Could you check a few things on this model? Use its own coordinates, in mm. A direction names the side the tool comes from. Give positions to 0.01 mm unless a question says otherwise; leave off trailing zeros. Write each loop counter-clockwise with the first axis right and the second up, starting at its lowest first coordinate (ties: lowest second). Pieces come first, ordered by that corner, then holes. Notation, with made-up numbers: (-2.75, 38) -> (10.25, 38) arc R16 ccw to (10.25, 64) -> close; hole circle Ø5 at (-9, 2.25). An arc over 180 degrees is marked (long way). One line per question, with ' | ' between items.
from build123d import *

# Parameters (mm, degrees)
F0_W     = 5
F0_H     = 5
F1_DEPTH = 5
F0_W_2   = 45
F0_W_3   = 40
F0_H_2   = 40
F2_DEPTH = 1


# Not quite as in the source:
# - a feature of the source that left no trace in its solid (it failed there, or was rolled back) is left out


with BuildPart() as f1:
    # F0 (on Top) → F1 (new body)
    with BuildSketch(Plane.XY):
        with Locations((-47.5, 45)):
            Rectangle(F0_W, F0_H)
    extrude(amount=F1_DEPTH)



with BuildPart() as f1b:
    # F0 (on Top) → F1, piece 2 (new body)
    with BuildSketch(Plane.XY):
        with Locations((-47.5, 0)):
            Rectangle(F0_W, F0_H)
    extrude(amount=F1_DEPTH)


with BuildPart() as f1c:
    # F0 (on Top) → F1, piece 3 (new body)
    with BuildSketch(Plane.XY):
        with Locations((-2.5, 0)):
            Rectangle(F0_W, F0_H)
    extrude(amount=F1_DEPTH)


with BuildPart() as f1d:
    # F0 (on Top) → F1, piece 4 (new body)
    with BuildSketch(Plane.XY):
        with Locations((47.5, 0)):
            Rectangle(F0_W, F0_H)
    extrude(amount=F1_DEPTH)


with BuildPart() as f1_1:
    add(f1.part)

    add(f1b.part)  # F2 merges F1b

    add(f1c.part)  # F2 merges F1c

    add(f1d.part)  # F2 merges F1d
    # F0 (on Top) → F2 (join)
    with BuildSketch(Plane.XY):
        with Locations((47.5, 0)):
            Rectangle(F0_W, F0_H)
        with Locations((22.5, 0)):
            Rectangle(F0_W_2, F0_H)
        with Locations((-2.5, 0)):
            Rectangle(F0_W, F0_H)
        with Locations((-25, 0)):
            Rectangle(F0_W_3, F0_H)
        with Locations((-47.5, 0)):
            Rectangle(F0_W, F0_H)
        with Locations((-47.5, 22.5)):
            Rectangle(F0_W, F0_H_2)
        with Locations((-47.5, 45)):
            Rectangle(F0_W, F0_H)
    extrude(amount=F2_DEPTH)


solid = f1_1.part
Q1. Imagine slicing it at A-A on z = 2.05. Please give me the cut outline in (x, y).
Answer below:
outline: (-50, -2.5) -> (-45, -2.5) -> (-45, 2.5) -> (-50, 2.5) -> close; (-50, 42.5) -> (-45, 42.5) -> (-45, 47.5) -> (-50, 47.5) -> close; (-5, -2.5) -> (0, -2.5) -> (0, 2.5) -> (-5, 2.5) -> close; (45, -2.5) -> (50, -2.5) -> (50, 2.5) -> (45, 2.5) -> close
Q2. Imagine slicing it at B-B on x = 7. Please give me the cut outline in (y, z), and give its area (3 significant figures).
Answer below:
outline: (-2.5, 0) -> (2.5, 0) -> (2.5, 1) -> (-2.5, 1) -> close | area: 5.00 mm^2
Q3. If we mould it in two halves opening along X, with no side actions, what happens to faces 1 (the flat face through (50, 0, 2)), 2 (the flat face through (-48, 2.5, 3)), 3 (the flat face through (-45, 0, 3))? For each: +X half, -X half, draft (parallel to the pull), parting line (faces both ways), or undercut.
Answer below:
face 1: +X half | face 2: draft | face 3: undercut
Q4. Imagine slicing it at C-C on y = 35.5. Please give me the cut outline in (x, z), and give its area (3 significant figures).
Answer below:
outline: (-50, 0) -> (-45, 0) -> (-45, 1) -> (-50, 1) -> close | area: 5.00 mm^2
Q5. If I drill on line 1 along X through (y, z) = (43, 2.5); line 2 along Z through (x, y) = (-29, 0.5); line 3 along Y through (x, z) = (-32, 0.5), over which ranges is the centre line in solid material (lowest first)?
Answer below:
line 1: x = -50 to -45 | line 2: z = 0 to 1 | line 3: y = -2.5 to 2.5
Q6. Will these pins go through, and if not, where does the flat tip stop? pin 1 (5.5 mm diameter, centred on x = 24, y = 0.5, fed in from +Z); pin 2 (2.5 mm diameter, centred on y = 21, z = 3, fed in from +X); pin 3 (1.5 mm diameter, centred on x = -5, z = 3, fed in from +Y).
Answer below:
pin 1: stops at z = 1 | pin 2: passes through | pin 3: stops at y = 2.5
Q7. On a 3-axis mill with a long thin cutter (end or side, diameter ignored), from which of +Z, -Z, +X, -X, +Y, -Y can I reach the whole of each face in a straight line? I mean faces 4 (the flat face through (-11.8, -2.5, 0.8)), 5 (the flat face through (-48, 23, 1)), 6 (the flat face through (-45, 31.6, 0.8)), 7 (the flat face through (-48, 0, 5)), 8 (the flat face through (22, 0, 1)). Say none if no direction works.
Answer below:
face 4: +Z, -Z, +X, -X, -Y | face 5: +Z, +X, -X | face 6: +Z, -Z, +X, +Y | face 7: +Z, +X, -X, +Y, -Y | face 8: +Z, +Y, -Y
